from build123d import *

# Parameters (mm, degrees)
SKETCH_1_R      = 1.5
EXTRUDE_1_DEPTH = 2


with BuildPart() as part:
    # 草图1 → 凸台-拉伸1 (new body)
    with BuildSketch(Plane.XY):
        with BuildLine():
            Line((24.667061038, -23.701524127), (24.667061038, 17.348475873))
            Line((24.667061038, 17.348475873), (-5.837728854, 17.348475873))
            ThreePointArc((-5.837728854, 17.348475873), (-12.908796666, 14.419543685), (-15.837728854, 7.348475873))
            ThreePointArc((-15.837728854, 7.348475873), (-20.286537867, -3.391899182), (-15.837728854, -14.132274238))
            Line((-15.837728854, -14.132274238), (-15.837728854, -36.151614729))
            Line((-15.837728854, -36.151614729), (48.322917805, -91.01542846))
            Line((48.322917805, -91.01542846), (58.385554114, -91.01542846))
            Line((58.385554114, -91.01542846), (58.385554114, -77.195903488))
            ThreePointArc((58.385554114, -77.195903488), (66.817061038, -65.025083014), (58.385554114, -52.85426254))
            Line((58.385554114, -52.85426254), (58.385554114, -41.837165292))
            Line((58.385554114, -41.837165292), (58.385554114, -36.151614729))
            Line((58.385554114, -36.151614729), (68.385554114, -36.151614729))
            Line((68.385554114, -36.151614729), (68.385554114, -27.701524127))
            Line((68.385554114, -27.701524127), (58.385554114, -27.701524127))
            Line((58.385554114, -27.701524127), (28.667061038, -27.701524127))
            ThreePointArc((28.667061038, -27.701524127), (25.838633913, -26.529951252), (24.667061038, -23.701524127))
        make_face()
        with Locations((6.667061038, -41.688027493)):
            Circle(SKETCH_1_R, mode=Mode.SUBTRACT)
        with BuildLine():
            Line((20.667061038, -54.125083014), (20.667061038, -45.925083014))
            Line((20.667061038, -45.925083014), (22.967061038, -45.925083014))
            Line((22.967061038, -45.925083014), (22.967061038, -54.125083014))
            ThreePointArc((22.967061038, -54.125083014), (21.817061038, -54.601428611), (20.667061038, -54.125083014))
        make_face(mode=Mode.SUBTRACT)
        with BuildLine():
            Line((52.717061038, -84.125083014), (52.717061038, -75.925083014))
            ThreePointArc((52.717061038, -75.925083014), (53.817061038, -75.469448095), (54.917061038, -75.925083014))
            Line((54.917061038, -75.925083014), (54.917061038, -84.125083014))
            Line((54.917061038, -84.125083014), (52.717061038, -84.125083014))
        make_face(mode=Mode.SUBTRACT)
        with Locations((58.385554114, -71.110493251)):
            Circle(SKETCH_1_R, mode=Mode.SUBTRACT)
        with Locations((58.385554114, -58.939672777)):
            Circle(SKETCH_1_R, mode=Mode.SUBTRACT)
        with BuildLine():
            Line((52.717061038, -54.125083014), (52.717061038, -45.925083014))
            Line((52.717061038, -45.925083014), (54.917061038, -45.925083014))
            Line((54.917061038, -45.925083014), (54.917061038, -54.125083014))
            ThreePointArc((54.917061038, -54.125083014), (53.817061038, -54.580717932), (52.717061038, -54.125083014))
        make_face(mode=Mode.SUBTRACT)
        with BuildLine():
            Line((-9.532938962, -29.250971973), (-9.532938962, -21.050971973))
            ThreePointArc((-9.532938962, -21.050971973), (-8.432938962, -20.595337054), (-7.332938962, -21.050971973))
            Line((-7.332938962, -21.050971973), (-7.332938962, -29.250971973))
            Line((-7.332938962, -29.250971973), (-9.532938962, -29.250971973))
        make_face(mode=Mode.SUBTRACT)
        with Locations((6.667061038, -20.300971973)):
            Circle(SKETCH_1_R, mode=Mode.SUBTRACT)
        with Locations((-15.837728854, -3.391899182)):
            Circle(SKETCH_1_R, mode=Mode.SUBTRACT)
        with BuildLine():
            Line((-9.532938962, 0.749028027), (-9.532938962, 8.949028027))
            Line((-9.532938962, 8.949028027), (-7.332938962, 8.949028027))
            Line((-7.332938962, 8.949028027), (-7.332938962, 0.749028027))
            ThreePointArc((-7.332938962, 0.749028027), (-8.432938962, 0.293393109), (-9.532938962, 0.749028027))
        make_face(mode=Mode.SUBTRACT)
        with Locations((6.667061038, -2.650971973)):
            Circle(SKETCH_1_R, mode=Mode.SUBTRACT)
        with BuildLine():
            Line((20.667061038, -11.350971973), (20.667061038, -6.050971973))
            ThreePointArc((20.667061038, -6.050971973), (21.817061038, -5.574626376), (22.967061038, -6.050971973))
            Line((22.967061038, -6.050971973), (22.967061038, -11.350971973))
            Line((22.967061038, -11.350971973), (20.667061038, -11.350971973))
        make_face(mode=Mode.SUBTRACT)
        with BuildLine():
            Line((20.667061038, 3.649028027), (20.667061038, 8.949028027))
            Line((20.667061038, 8.949028027), (22.967061038, 8.949028027))
            Line((22.967061038, 8.949028027), (22.967061038, 3.649028027))
            ThreePointArc((22.967061038, 3.649028027), (21.817061038, 3.172682431), (20.667061038, 3.649028027))
        make_face(mode=Mode.SUBTRACT)
    extrude(amount=EXTRUDE_1_DEPTH)


solid = part.part
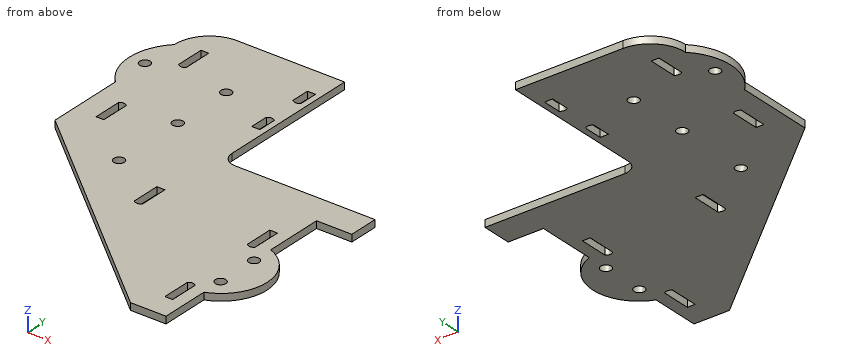
Read the model definition and answer for the solid it produces. Units are mm, in the model's axes. Give positions to 0.01 mm unless a question says otherwise; leave off trailing zeros. Write each loop counter-clockwise with the first axis right and the second up, starting at its lowest first coordinate (ties: lowest second). Pieces come first, ordered by that corner, then holes. Notation, with made-up numbers: (-33.75, 71) - (17.25, 71) arc R7 cw to (17.25, 80) - close; hole circle Ø8 at (-36.5, -4). An arc over 180 degrees is marked (long way). Use CSV: the item, a comma, the result in double quotes. Start each with the question number.
Item 1: The part is cut by section B-B, the plane y = 5.5. Give the vertices of the cut face in (x, z).
Item 2: Flat-ended cylindrical pins translate along their axes: P1, Ø1, axis at x = 53.5, z = 1, coming from the +Y side; P2, Ø1, axis at y = -7.5, z = 1.5, coming from the -X side; P3, Ø1, axis at y = -25.5, z = 1.5, coming from the -X side. Find the tip coordinate at first contact, or state that the pin passes through.
Item 3: The part is cut by section D-D, the plane x = 51.5. Give the vertices of the cut face in (y, z).
Item 4: The part is cut by section C-C, the plane z = 0.5. Count the separate pieces of the cut face and the enclosed holes in it, and give its area (3 significant figures).
Item 5: The part is cut by section A-A, the plane y = -82. Give the vertices of the cut face in (x, z), and give its area (3 significant figures).
Item 6: Consider line 1 (Y direction, x = -9.5, z = 1.1); line 2 (X direction, y = -20.5, z = 1.2); line 3 (X direction, y = -47.5, z = 1.8). Determine where each line is inside the solid, lowest interval first.
Taken from the geometry:
1,outline,"(-17.41, 0) - (-9.53, 0) - (-9.53, 2) - (-17.41, 2) - close; (-7.33, 0) - (20.67, 0) - (20.67, 2) - (-7.33, 2) - close; (22.97, 0) - (24.67, 0) - (24.67, 2) - (22.97, 2) - close"
2,P1,"y = -27.7"
2,P2,"x = -19.85"
2,P3,"x = -15.84"
3,outline,"(-91.02, 0) - (-27.7, 0) - (-27.7, 2) - (-91.02, 2) - close"
4,separate pieces,"1"
4,enclosed holes,"13"
4,area,"4,880 mm2"
5,outline,"(37.78, 0) - (52.72, 0) - (52.72, 2) - (37.78, 2) - close; (54.92, 0) - (58.39, 0) - (58.39, 2) - (54.92, 2) - close"
5,area,"36.8 mm2"
6,line 1,"-41.57 to -29.25, -21.02 to 0.72, 8.95 to 16.65"
6,line 2,"-15.84 to 5.18, 8.15 to 24.67"
6,line 3,"-2.57 to 20.67, 22.97 to 52.72, 54.92 to 58.39"
